Autodesk Inventor part; units mm, degrees
ref_plane "YZ Plane" through (0, 0, 0) normal (1, 0, 0) x (0, 1, 0)
ref_plane "XZ Plane" through (0, 0, 0) normal (0, 1, 0) x (-1, 0, 0)
ref_plane "XY Plane" through (0, 0, 0) normal (0, 0, 1) x (1, 0, 0)
sketch "Esboço1" plane through (0, 0, 0) normal (0, 1, 0) x (-1, 0, 0)
  line L0 (0, 0) -> (200, 0)
  line L1 (200, 0) -> (200, -200)
  line L2 (200, -200) -> (0, -200)
  line L3 (0, -200) -> (0, 0)
  dimension "d0" = 200
  dimension "d1" = 200
extrude "Extrusão1" add sketch "Esboço1" along normal blind 3.0625
sketch "Esboço2" plane through (0, 3.0625, 0) normal (0, 1, 0) x (1, 0, 0)
  line L0 (0, 0) -> (0, 200)
  line L1 (-200, 0) -> (0, 0)
  line L2 (-200, 200) -> (-200, 0)
  line L3 (0, 200) -> (-200, 200)
  point P0 (-10, 10)
  point P1 (-190, 10)
  point P2 (-190, 190)
  point P3 (-10, 190)
  dimension "d4" = 10
  dimension "d5" = 10
  dimension "d6" = 10
  dimension "d7" = 10
  dimension "d8" = 10
  dimension "d9" = 10
  dimension "d10" = 10
  dimension "d11" = 10
  dimension "d34" = 200
  dimension "d35" = 200
hole "Furo1" at (-10, 3.0625, -10) at (-190, 3.0625, -10) at (-190, 3.0625, -190) at (-10, 3.0625, -190) direction (0, -1, 0) diameter 5 end through all
sketch "Esboço3" plane through (0, 3.0625, 0) normal (0, 1, 0) x (1, 0, 0)
  line L0 (-200, 200) -> (-200, 0)
  line L1 (-200, 0) -> (0, 0)
  line L2 (0, 0) -> (0, 200)
  line L3 (0, 200) -> (-200, 200)
  point P0 (-32.5, 100)
  point P1 (-167.5, 100)
  dimension "d22" = 135
  dimension "d46" = 200
  dimension "d49" = 100
  dimension "d50" = 0
  dimension "d51" = 32.5
hole "Furo2" at (-32.5, 3.0625, -100) at (-167.5, 3.0625, -100) direction (0, -1, 0) diameter 5 depth 3.0625
equation "\"d17\" = Espessura"
equation "\"d32\" = Espessura"
equation "\"Raio_vergadura\" = Espessura"
equation "\"Largura_alívio_de_vergadura\" = Espessura"
equation "\"Profundidade_alívio_de_vergadura\" = 0.5 * Espessura"
equation "\"Tamanho_alívio_de_dobra\" = 4 * Espessura"
equation "\"Remanescente_mínimo\" = 2 * Espessura"
equation "\"Raiodetransição\" = Raio_vergadura"
equation "\"Tamanho_de_raio_de_Jacobi\" = Raio_vergadura"
equation "\"TamanhoFolga\" = Espessura"
properties part number "Base de apoio" material "Aço inoxidável"
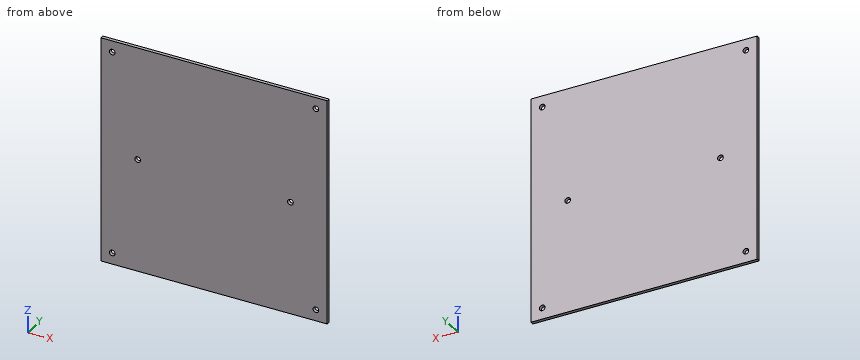
Can you work these out from the model? Positions are in its coordinate system, mm. Coordinates: 2 decimals unless noted, no trailing zeros. Order: outer loops, then holes, each group sorted by start corner. A loop starts at its lowest first (then second) coordinate and runs counter-clockwise, first axis right, second up. Notation, with made-up numbers: (48, -13) - (93, -13) arc R18 ccw to (93, 13) - close; hole circle Ø2 at (-38, -38). An arc over 180 degrees is marked (long way). Answer as a JSON object with one key per item and string values. Group by question number.
Q1. I need wall thicknesses on line 1 (Z direction, x = -190, y = 0.9); line 2 (Z direction, x = -32, y = 1.05). Which ranges of each line are inside material? Lowest first, please. Write a range as from..to.
Q2. Imagine slicing it at A-A (z = -100). Please give me the cut outline in (x, y), and give its area (3 significant figures).
Q3. Imagine slicing it at B-B (x = -167.5). Please give me the cut outline in (y, z).
Q4. Will this pin go through, and if not, where does the flat tip stop? P1, Ø4.5, axis at x = -10, z = -10, coming from the -Y side.
Determined:
{
 "1": {"line 1": "z = -200..-192.5, -187.5..-12.5, -7.5..0", "line 2": "z = -200..-102.45, -97.55..0"},
 "2": {"outline": "(-200, 0) - (-170, 0) - (-170, 3.06) - (-200, 3.06) - close; (-165, 0) - (-35, 0) - (-35, 3.06) - (-165, 3.06) - close; (-30, 0) - (0, 0) - (0, 3.06) - (-30, 3.06) - close", "area": "582 mm2"},
 "3": {"outline": "(0, -200) - (3.06, -200) - (3.06, -102.5) - (0, -102.5) - close; (0, -97.5) - (3.06, -97.5) - (3.06, 0) - (0, 0) - close"},
 "4": {"P1": "passes through"}
}
